Geometry check sheet. Reference: the model listing, model coordinates, mm. Coordinates: 2 decimals unless noted, no trailing zeros.
Autodesk Inventor part; units mm, degrees
ref_plane "YZ Plane" through (0, 0, 0) normal (1, 0, 0) x (0, 1, 0)
ref_plane "XZ Plane" through (0, 0, 0) normal (0, 1, 0) x (-1, 0, 0)
ref_plane "XY Plane" through (0, 0, 0) normal (0, 0, 1) x (1, 0, 0)
sketch "Sketch1" plane through (0, 0, 0) normal (0, 0, 1) x (1, 0, 0)
  line L0 (-16.75, 16.75) -> (16.75, 16.75)
  line L1 (16.75, 16.75) -> (16.75, -16.75)
  line L2 (16.75, -16.75) -> (-16.75, -16.75)
  line L3 (-16.75, -16.75) -> (-16.75, 16.75)
  line L4 (-16.75, 16.75) -> (16.75, -16.75) construction
  line L5 (16.75, 16.75) -> (-16.75, -16.75) construction
  point P0 (0, 0)
  dimension "d0" = 33.5
  dimension "d1" = 33.5
extrude "Extrusion1" add sketch "Sketch1" along normal mid plane 50.5
sketch "Sketch2" plane through (0, 0, 25.25) normal (0, 0, 1) x (1, 0, 0)
  line L0 (-11.75, 11.75) -> (11.75, 11.75)
  line L1 (11.75, 11.75) -> (11.75, -11.75)
  line L2 (11.75, -11.75) -> (-11.75, -11.75)
  line L3 (-11.75, -11.75) -> (-11.75, 11.75)
  line L4 (-11.75, 11.75) -> (11.75, -11.75) construction
  line L5 (11.75, 11.75) -> (-11.75, -11.75) construction
  line L6 (16.75, 16.75) -> (-16.75, 16.75)
  line L7 (16.75, -16.75) -> (16.75, 16.75)
  point P0 (0, 0)
  dimension "d4" = 5
  dimension "d5" = 5
extrude "Extrusion2" cut sketch "Sketch2" against normal blind 1
sketch "Sketch3" plane through (0, 0, -25.25) normal (0, 0, -1) x (-1, 0, 0)
  point P0 (0, 0)
properties part number "acrylicpmt"
1. Thickness scan on line 1 along Z through (x, y) = (-6.5, 5). Record the ranges inside material, lowest first.
Computed values:
line 1: z = -25.25 to 24.25
2. Draft check along X on faces 1 (the flat face through (-16.75, 0, 0)), 2 (the flat face through (0, 0, 24.25)), 3 (the flat face through (0, -16.75, 0)). Enter one of: released by +X, released by -X, zero draft, split by the parting line, or undercut.
Computed values:
face 1: released by -X
face 2: undercut
face 3: zero draft
3. Gauge pin test, flat end, axial feed: pin 1 Ø6 at (x, y) = (7, -8) entering from +Z. Record the tip position at first contact, or that the pin passes through.
Computed values:
pin 1: stops at z = 24.25
